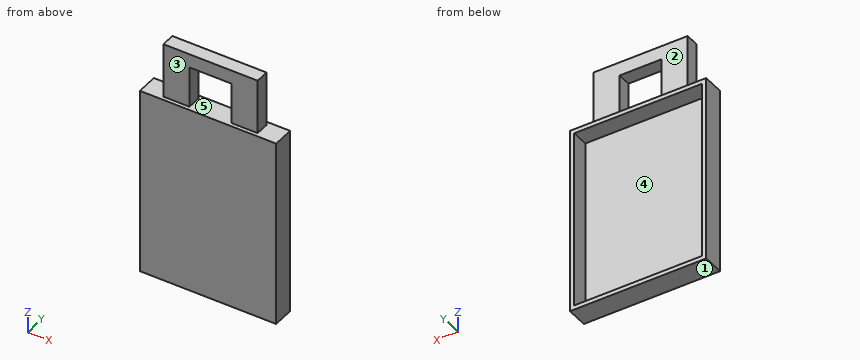
```python
from build123d import *

# Parameters (mm, degrees)
SKETCH1_W           = 159
SKETCH1_H           = 25
BOSS_EXTRUDE1_DEPTH = 220
SKETCH2_W           = 149
SKETCH2_H           = 210
CUT_EXTRUDE1_DEPTH  = 20
SKETCH3_W           = 30.44
SKETCH3_H           = 16
BOSS_EXTRUDE2_DEPTH = 64
BOSS_EXTRUDE3_REACH = 106.03
SKETCH4_W           = 16
SKETCH4_H           = 16


with BuildPart() as part:
    # Sketch1 → Boss-Extrude1 (new body)
    with BuildSketch(Plane.XY):
        with Locations((0, 12.5)):
            Rectangle(SKETCH1_W, SKETCH1_H)
    extrude(amount=BOSS_EXTRUDE1_DEPTH)

    # Sketch2 → Cut-Extrude1 (cut)
    with BuildSketch(Plane(origin=(0, 25, 0), x_dir=(1, 0, 0), z_dir=(0, 1, 0))):
        with Locations((0, -110)):
            Rectangle(SKETCH2_W, SKETCH2_H)
    extrude(amount=-CUT_EXTRUDE1_DEPTH, mode=Mode.SUBTRACT)

    # Sketch3 → Boss-Extrude2 (add)
    with BuildSketch(Plane.XY.offset(220)):
        with Locations((-39.75, 12.5)):
            Rectangle(SKETCH3_W, SKETCH3_H)
    boss_extrude2 = extrude(amount=BOSS_EXTRUDE2_DEPTH)

    # Mirror1: Boss-Extrude2 across plane
    add(boss_extrude2.mirror(Plane(origin=(0, 0, 0), x_dir=(0, 0, 1), z_dir=(1, 0, 0))))

    # Sketch4 → Boss-Extrude3 (add, up to next)
    with BuildSketch(Plane(origin=(-24.53, 0, 0), x_dir=(0, 0, -1), z_dir=(1, 0, 0)), mode=Mode.PRIVATE) as boss_extrude3_sk1:
        with Locations((-276, 12.5)):
            Rectangle(SKETCH4_W, SKETCH4_H)
    boss_extrude3_tool1 = extrude(boss_extrude3_sk1.sketch, amount=BOSS_EXTRUDE3_REACH, mode=Mode.PRIVATE) - part.part
    add(boss_extrude3_tool1.solids().sort_by_distance((-24.53, 12.5, 276))[0])


solid = part.part
```
Can you work these out from the model? Positions are in its coordinate system, mm. Face numbers are marked on the shaded views. A direction names the side the tool comes from. Give positions to 0.01 mm unless a question says otherwise; leave off trailing zeros. Loops run counter-clockwise (first coordinate to the right, second up) from the corner with the lowest first, then second, coordinate; pieces in that order, holes last. Notation, with made-up numbers: M 68,-20.5 L 117,-20.5 A24 cw 117,5.5 Z; hole C 12,32.25 d8. An arc over 180 degrees is marked long. Answer in a Markdown table with one row per item.
1. Suppose I cut it at A-A on y = 8. Write out the boundary of the cut face in (x, z).
Taken from the geometry:
| item | result |
|---|---|
| outline | M -79.5,0 L 79.5,0 L 79.5,220 L 54.97,220 L 54.97,284 L -54.97,284 L -54.97,220 L -79.5,220 Z; hole M -74.5,5 L 74.5,5 L 74.5,215 L -74.5,215 Z; hole M -24.53,220 L 24.53,220 L 24.53,268 L -24.53,268 Z |
2. Suppose I cut it at D-D on x = -59. Write out the boundary of the cut face in (y, z), plus the area to 3 significant figures.
Taken from the geometry:
| item | result |
|---|---|
| outline | M 0,0 L 25,0 L 25,5 L 5,5 L 5,215 L 25,215 L 25,220 L 0,220 Z |
| area | 1,300 mm² |
3. Suppose I cut it at C-C on z = 133. Write out the boundary of the cut face in (x, y), plus the area to 3 significant figures.
Taken from the geometry:
| item | result |
|---|---|
| outline | M -79.5,0 L 79.5,0 L 79.5,25 L 74.5,25 L 74.5,5 L -74.5,5 L -74.5,25 L -79.5,25 Z |
| area | 995 mm² |
4. Which directions (+Z, -Z, +X, -X, +Y, -Y) give clear straight access to the entire face, cutting with the end or side of a thin tool? Please do the marked faces 1 and 2.
Taken from the geometry:
| item | result |
|---|---|
| face 1 | -Z, +X, -X, +Y, -Y |
| face 2 | +Z, +X, -X, +Y |
5. Thinking about a two-plate mould opening in X: for the marked faces 3, 4 and 5, which applies, released by +X, released by -X, zero draft, split by the parting line, or undercut?
Taken from the geometry:
| item | result |
|---|---|
| face 3 | zero draft |
| face 4 | undercut |
| face 5 | undercut |
6. For pin 1 Ø5 at (x, y) = (-0.5, 14) entering from -Z; pin 2 Ø8 at (y, z) = (9, 261) entering from +X; pin 3 Ø3 at (x, y) = (58, 15.5) entering from +Z; pin 4 Ø13 at (y, z) = (16, 240) entering from -X, each with a flat end and sliding along its axis, tell me the tip position at first contact or that it passes through.
Taken from the geometry:
| item | result |
|---|---|
| pin 1 | stops at z = 0 |
| pin 2 | stops at x = 54.97 |
| pin 3 | stops at z = 220 |
| pin 4 | stops at x = -54.97 |
7. If I drill on line 1 along Z through (x, y) = (-10, 12.5); line 2 along X through (y, z) = (24, 120.5); line 3 along Z through (x, y) = (25.5, 10.5), over which ranges is the centre line in solid material (lowest first)?
Taken from the geometry:
| item | result |
|---|---|
| line 1 | z = 0 to 5, 215 to 220, 268 to 284 |
| line 2 | x = -79.5 to -74.5, 74.5 to 79.5 |
| line 3 | z = 0 to 5, 215 to 284 |
8. Suppose I cut it at B-B on x = -7.5. Write out the boundary of the cut face in (y, z), plus the area to 3 significant figures.
Taken from the geometry:
| item | result |
|---|---|
| outline | M 0,0 L 25,0 L 25,5 L 5,5 L 5,215 L 25,215 L 25,220 L 0,220 Z; M 4.5,268 L 20.5,268 L 20.5,284 L 4.5,284 Z |
| area | 1,560 mm² |
